```python
from build123d import *

# Parameters (mm, degrees)
SKETCH2_R          = 1.5
CUT_EXTRUDE1_DEPTH = 4


with BuildPart() as part:
    # Sketch1 → Revolve1 (revolve)
    with BuildSketch(Plane.XY, mode=Mode.PRIVATE) as revolve1_sk:
        Polygon((0, 30), (2.5, 30), (2.5, 18), (14, 18), (14, 8), (5.5, 8), (5.5, 4), (11.5, 4), (11.5, 0), (0, 0), align=None)
    revolve(revolve1_sk.sketch.rotate(Axis((0, 0, 0), (0, 1, 0)), 90), axis=Axis((0, 0, 0), (0, 1, 0)))

    # Sketch2 → Cut-Extrude1 (cut)
    with BuildSketch(Plane.XZ):
        with Locations(Location((0, 8, 0), (0, 0, 270))):
            Circle(SKETCH2_R)
        with Locations(Location((8, 0, 0), (0, 0, 270))):
            Circle(SKETCH2_R)
        with Locations(Location((0, -8, 0), (0, 0, 270))):
            Circle(SKETCH2_R)
        with Locations(Location((-8, 0, 0), (0, 0, 270))):
            Circle(SKETCH2_R)
    extrude(amount=-CUT_EXTRUDE1_DEPTH, mode=Mode.SUBTRACT)


solid = part.part
```
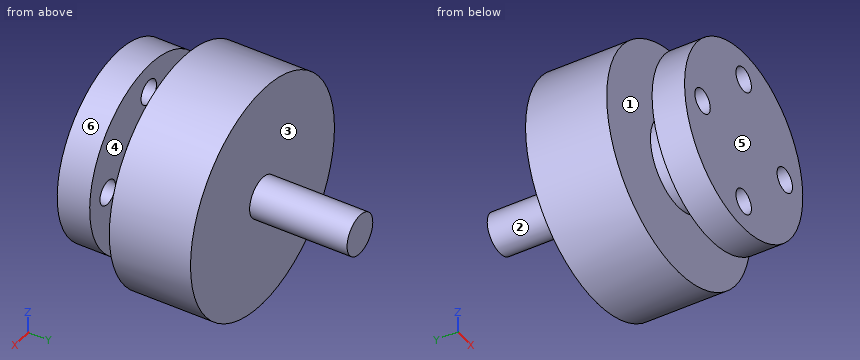
The listing builds one solid part. Answer for the finished solid, in the listing's coordinates (mm). Face numbers are marked on the shaded views. A direction names the side the tool comes from. Give positions to 0.01 mm unless a question says otherwise; leave off trailing zeros. Write each loop counter-clockwise with the first axis right and the second up, starting at its lowest first coordinate (ties: lowest second). Pieces come first, ordered by that corner, then holes. Notation, with made-up numbers: (-25.5, -35) - (13.5, -35) arc R9 cw to (13.5, -29) - close; hole circle Ø2 at (-13.5, 10). An arc over 180 degrees is marked (long way). Use one line per item in the form item = value. Start each with the question number.
1) Find section C-C on x = 0. Determine the outline of the cut face in (y, z), plus the area to 3 significant figures.
2) Find section A-A on z = 0. Determine the outline of the cut face in (x, y), plus the area to 3 significant figures.
3) The mould has two halves that part along Y. Classify the marked faces 1, 2 and 3: pulls with the +Y half, pulls with the -Y half, needs draft (parallel to the pull), parting line crosses it, or undercut.
4) Consider line 1 along X through (y, z) = (1.35, 0); line 2 along Y through (x, z) = (-7.25, -8.5); line 3 along Y through (x, z) = (1.25, 12.25). Determine where each line is inside the solid, lowest interval first. Write a range as from..to.
5) Flat-ended cylindrical pins translate along their axes: pin 1 Ø2.5 at (x, z) = (0, 8) entering from -Y; pin 2 Ø5 at (x, z) = (0, -8) entering from +Y; pin 3 Ø4 at (x, z) = (4.5, -10.5) entering from -Y; pin 4 Ø12 at (x, y) = (-9, 5) entering from +Z. Find the tip coordinate at first contact, or state that the pin passes through.
6) Find section D-D on z = -7.5. Determine the outline of the cut face in (x, y).
7) Find section B-B on y = 3.5. Determine the outline of the cut face in (x, z), plus the area to 3 significant figures.
8) A tool of negligible diameter and unlimited length cuts with its end or side. For the marked faces 4, 5 and 6, from which of +Z, -Z, +X, -X, +Y, -Y can it reach the whole face along a straight path? Write none if from no direction.
Geometry results:
q1.outline = (0, -11.5) - (4, -11.5) - (4, -9.5) - (0, -9.5) - close; (0, -6.5) - (4, -6.5) - (4, -5.5) - (8, -5.5) - (8, -14) - (18, -14) - (18, -2.5) - (30, -2.5) - (30, 2.5) - (18, 2.5) - (18, 14) - (8, 14) - (8, 5.5) - (4, 5.5) - (4, 6.5) - (0, 6.5) - close; (0, 9.5) - (4, 9.5) - (4, 11.5) - (0, 11.5) - close
q1.area = 452 mm2
q2.outline = (-14, 8) - (-5.5, 8) - (-5.5, 4) - (-6.5, 4) - (-6.5, 0) - (6.5, 0) - (6.5, 4) - (5.5, 4) - (5.5, 8) - (14, 8) - (14, 18) - (2.5, 18) - (2.5, 30) - (-2.5, 30) - (-2.5, 18) - (-14, 18) - close; (-11.5, 0) - (-9.5, 0) - (-9.5, 4) - (-11.5, 4) - close; (9.5, 0) - (11.5, 0) - (11.5, 4) - (9.5, 4) - close
q2.area = 452 mm2
q3.face_1 = undercut
q3.face_2 = needs draft
q3.face_3 = pulls with the +Y half
q4.line_1 = -11.5..-9.5, -6.5..6.5, 9.5..11.5
q4.line_2 = 0..4, 8..18
q4.line_3 = 8..18
q5.pin_1 = 8
q5.pin_2 = 18
q5.pin_3 = 0
q5.pin_4 = 13.47
q6.outline = (-11.82, 8) - (11.82, 8) - (11.82, 18) - (-11.82, 18) - close; (-8.72, 0) - (-1.41, 0) - (-1.41, 4) - (-8.72, 4) - close; (1.41, 0) - (8.72, 0) - (8.72, 4) - (1.41, 4) - close
q7.outline = circle Ø23 at (0, 0); hole circle Ø3 at (-8, 0); hole circle Ø3 at (0, -8); hole circle Ø3 at (0, 8); hole circle Ø3 at (8, 0)
q7.area = 387 mm2
q8.face_4 = none
q8.face_5 = +Z, -Z, +X, -X, -Y
q8.face_6 = -Y
